Geometry: see drawing. Coordinates: mm, zero at the bounding-box minimum. Give positions to 0.01 mm unless a question says otherwise; leave off trailing zeros. Write each loop counter-clockwise with the first axis right and the second up, starting at its lowest first coordinate (ties: lowest second). Pieces come first, ordered by that corner, then holes. Notation, with made-up numbers: (73.5, -16) - (83.5, -16) arc R10 ccw to (83.5, -10) - close; hole circle Ø3 at (0, 56). An arc over 180 degrees is marked (long way). Use a Markdown table: item, result. Add a question column.
1. Pin query (flat end, axial travel): pin 1 (12 mm diameter, centred on x = 17.5, y = 9.5, fed in from +Z); pin 2 (12 mm diameter, centred on x = 6.5, z = 20, fed in from -Y); pin 3 (8 mm diameter, centred on x = 17.5, y = 24.5, fed in from +Z). Return the tip coordinate at first contact, or that it passes through.
2. Section query D-D, the plane y = 28.25. Return loops of the section in (x, z).
3. Section query B-B, the plane y = 8.5. Return loops of the section in (x, z), plus the area to 3 significant figures.
4. Section query A-A, the plane x = 12.5. Count the separate pieces of the cut face and the enclosed holes in it, plus the area to 3 significant figures.
5. Material intervals for probe 1 along Z at (x, y) = (3.25, 16.75); probe 2 along Y at (x, z) = (4.5, 15); probe 3 along Y at (x, z) = (12.5, 2.1), sorted ascending.
6. Mould query, pull axis Y, two halves, no side actions, for the marked faces 1, 2 and 3. Classes: released by +Y, released by -Y, zero draft, split by the parting line, or undercut.
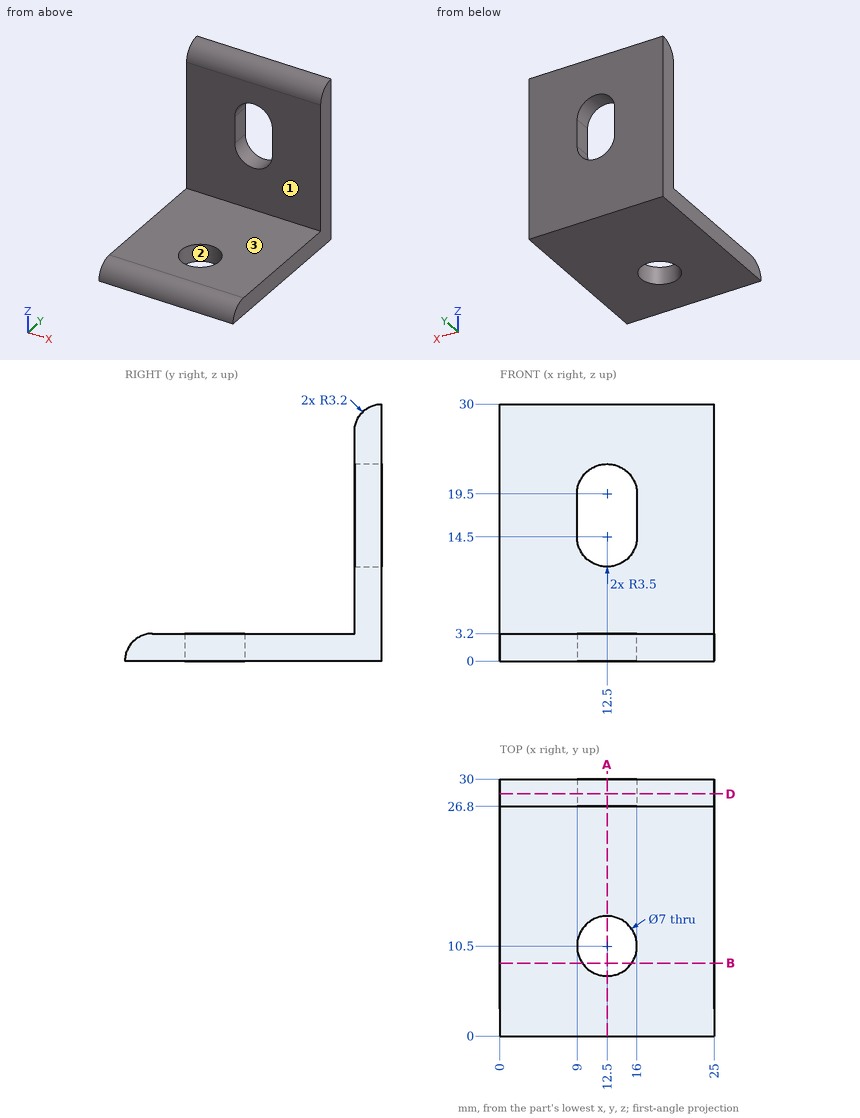
Result sheet:
| question | item | result |
|---|---|---|
| 1 | pin 1 | stops at z = 3.2 |
| 1 | pin 2 | stops at y = 26.8 |
| 1 | pin 3 | stops at z = 29.63 |
| 2 | outline | (0, 0) - (25, 0) - (25, 29.48) - (0, 29.48) - close; hole (9, 14.5) arc R3.5 ccw to (16, 14.5) - (16, 19.5) arc R3.5 ccw to (9, 19.5) - close |
| 3 | outline | (0, 0) - (9.63, 0) - (9.63, 3.2) - (0, 3.2) - close; (15.37, 0) - (25, 0) - (25, 3.2) - (15.37, 3.2) - close |
| 3 | area | 61.6 mm² |
| 4 | separate pieces | 3 |
| 4 | enclosed holes | 0 |
| 4 | area | 117 mm² |
| 5 | probe 1 | z = 0 to 3.2 |
| 5 | probe 2 | y = 26.8 to 30 |
| 5 | probe 3 | y = 0.79 to 7, 14 to 30 |
| 6 | face 1 | released by -Y |
| 6 | face 2 | undercut |
| 6 | face 3 | zero draft |
